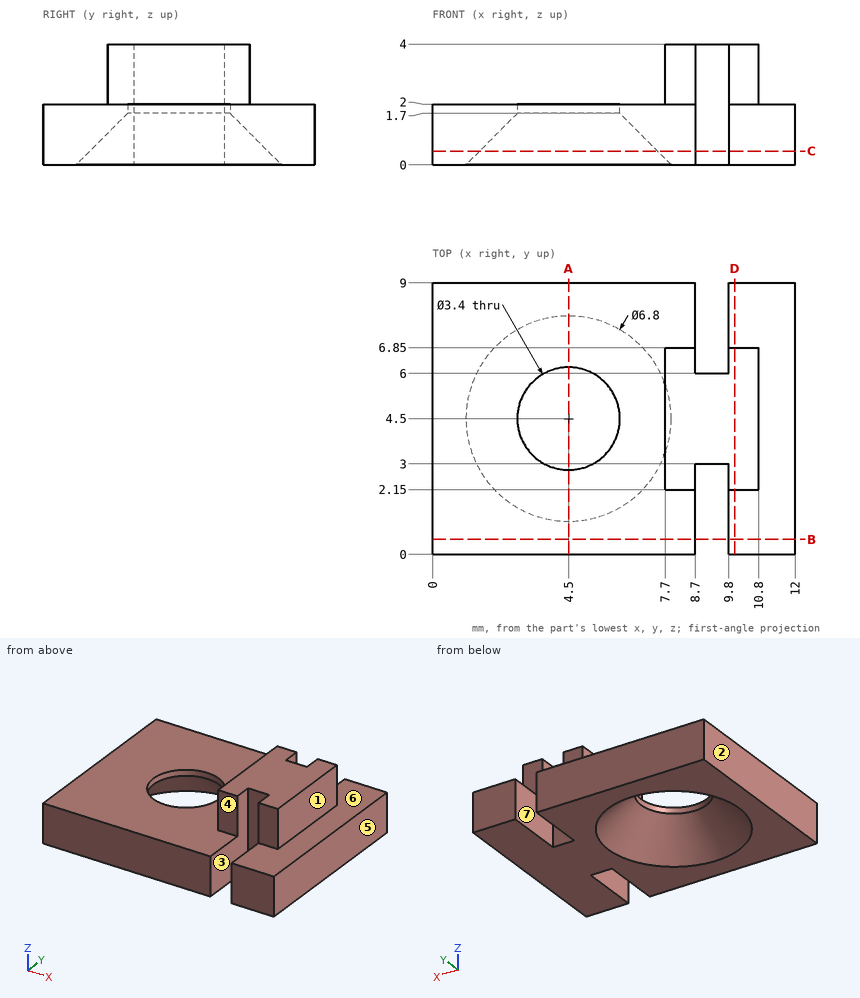
Here's the drawing with two shaded views (mm, measured from the low corner). I have some questions. A direction names the side the tool comes from. Give positions to 0.01 mm unless a question says otherwise; leave off trailing zeros. Loops run counter-clockwise (first coordinate to the right, second up) from the corner with the lowest first, then second, coordinate; pieces in that order, holes last. Notation, with made-up numbers: (32, 78.25) -> (51, 78.25) arc R12 cw to (51, 87.25) -> close; hole circle Ø8 at (-8.5, 56). An arc over 180 degrees is marked (long way). One line per item, written item: value.
Q1. I'm going to push flat-ended pins straight in: pin 1 Ø1 at (x, y) = (7.5, 2.5) entering from -Z; pin 2 Ø0.9 at (y, z) = (1.5, 3) entering from +X; pin 3 Ø0.8 at (x, z) = (8, 3) entering from +Y; pin 4 Ø1.6 at (y, z) = (5.5, 3.5) entering from -X. Where does each tip first touch, or does it pass through?
Answers follow:
pin 1: z = 0
pin 2: through
pin 3: y = 6.85
pin 4: x = 7.7
Q2. On a 3-axis mill with a long thin cutter (end or side, diameter ignored), from which of +Z, -Z, +X, -X, +Y, -Y can I reach the whole of each face in a straight line? I mean the marked faces 1, 2, 3 and 4. Say none if no direction works.
Answers follow:
face 1: +Z, +X, +Y, -Y
face 2: +Z, -Z, -X, +Y, -Y
face 3: +Z, -Z, -Y
face 4: +Z, +X, -X, -Y
Q3. If I drill on line 1 along X through (y, z) = (8.25, 0.7); line 2 along Y through (x, z) = (4.5, 1.9); line 3 along X through (y, z) = (6.25, 0.85), over which ranges is the centre line in solid material (lowest first)?
Answers follow:
line 1: 0 to 8.7, 9.8 to 12
line 2: 0 to 2.8, 6.2 to 9
line 3: 0 to 2.65, 6.35 to 8.7, 9.8 to 12
Q4. Suppose I cut it at C-C on z = 0.45. Please give me the cut outline in (x, y), then the cut area to 3 significant figures.
Answers follow:
outline: (0, 0) -> (8.7, 0) -> (8.7, 3) -> (9.8, 3) -> (9.8, 0) -> (12, 0) -> (12, 9) -> (9.8, 9) -> (9.8, 6) -> (8.7, 6) -> (8.7, 9) -> (0, 9) -> close; hole circle Ø5.9 at (4.5, 4.5)
area: 74.1 mm^2
Q5. Suppose I cut it at B-B on y = 0.5. Please give me the cut outline in (x, z).
Answers follow:
outline: (0, 0) -> (8.7, 0) -> (8.7, 2) -> (0, 2) -> close; (9.8, 0) -> (12, 0) -> (12, 2) -> (9.8, 2) -> close
Q6. Suppose I cut it at A-A on x = 4.5. Please give me the cut outline in (y, z).
Answers follow:
outline: (0, 0) -> (1.1, 0) -> (2.8, 1.7) -> (2.8, 2) -> (0, 2) -> close; (6.2, 1.7) -> (7.9, 0) -> (9, 0) -> (9, 2) -> (6.2, 2) -> close
Q7. Suppose I cut it at D-D on x = 10. Please give me the cut outline in (y, z).
Answers follow:
outline: (0, 0) -> (9, 0) -> (9, 2) -> (6.85, 2) -> (6.85, 4) -> (2.15, 4) -> (2.15, 2) -> (0, 2) -> close
Q8. We'd pull the mould along X, two halves only. Please class the marked faces 5, 6 and 7: pulls with the +X half, pulls with the -X half, needs draft (parallel to the pull), parting line crosses it, or undercut.
Answers follow:
face 5: pulls with the +X half
face 6: needs draft
face 7: undercut
